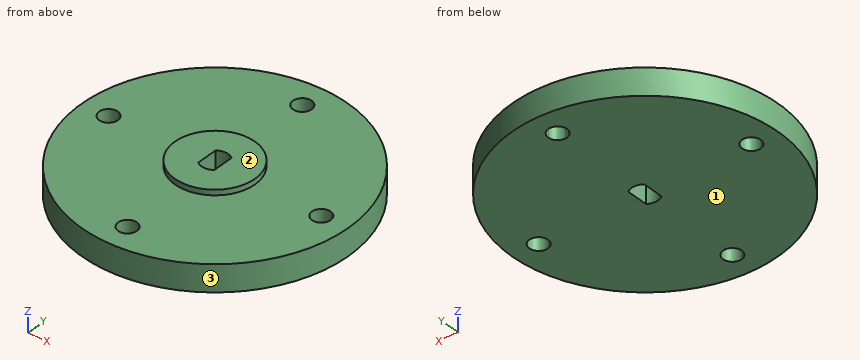
```python
from build123d import *

# Parameters (mm, degrees)
F0_R     = 7.5
F0_R_2   = 25
F1_DEPTH = 5
F2_DEPTH = 6
F3_R     = 1.75
F4_DEPTH = 5


with BuildPart() as f1:
    # F0 (on Top) → F1 (new body)
    with BuildSketch(Plane.XY):
        Circle(F0_R)
        with BuildLine():
            ThreePointArc((1.5, -2), (0, -2.5), (-1.5, -2))
            Line((-1.5, -2), (-1.5, 2))
            ThreePointArc((-1.5, 2), (0, 2.5), (1.5, 2))
            Line((1.5, 2), (1.5, -2))
        make_face(mode=Mode.SUBTRACT)
        Circle(F0_R_2)
        Circle(F0_R, mode=Mode.SUBTRACT)
    extrude(amount=F1_DEPTH)

    # F0 (on Top) → F2 (join)
    with BuildSketch(Plane.XY):
        Circle(F0_R)
        with BuildLine():
            ThreePointArc((1.5, -2), (0, -2.5), (-1.5, -2))
            Line((-1.5, -2), (-1.5, 2))
            ThreePointArc((-1.5, 2), (0, 2.5), (1.5, 2))
            Line((1.5, 2), (1.5, -2))
        make_face(mode=Mode.SUBTRACT)
    extrude(amount=F2_DEPTH)

    # F3 (on face) → F4 (cut)
    with BuildSketch(Plane.XY.offset(5)):
        with BuildLine():
            ThreePointArc((0, 18.25), (1.237437, 18.762563), (1.75, 20))
            ThreePointArc((1.75, 20), (-1.237437, 21.237437), (0, 18.25))
        make_face()
        with Locations((20, 0)):
            Circle(F3_R)
        with Locations((0, -20)):
            Circle(F3_R)
        with Locations((-20, 0)):
            Circle(F3_R)
    extrude(amount=-F4_DEPTH, mode=Mode.SUBTRACT)


solid = f1.part
```
Check sheet for the modelled part. Datum: model origin and axes. Units: mm. Face numbers are marked on the shaded views. Give positions to 0.01 mm unless a question says otherwise; leave off trailing zeros. Write each loop counter-clockwise with the first axis right and the second up, starting at its lowest first coordinate (ties: lowest second). Pieces come first, ordered by that corner, then holes.
Item 1: Draft check along Z on the marked faces 1, 2 and 3. Enter one of: released by +Z, released by -Z, zero draft, split by the parting line, or undercut.
Item 2: Scan lines: L1, parallel to Y at x = 0, z = 2.5; L2, parallel to Z at x = -5, y = 6.5; L3, parallel to X at y = 21.5, z = 2.4. Record each from-to range of solid material in increasing order.
Item 3: Cross-section at A-A (y = 0). Enter the section's corners in (x, z).
Item 4: Cross-section at B-B (x = -20). Enter the section's corners in (y, z).
Item 5: Cross-section at D-D (z = 1.1). Enter the section's corners in (x, y).
Item 6: Gauge pin test, flat ends, axial feed: pin 1 (1.5 mm diameter, centred on y = -8, z = 0.5, fed in from +X); pin 2 (4 mm diameter, centred on x = 0, y = -20, fed in from -Z); pin 3 (2 mm diameter, centred on x = 20, y = 0, fed in from -Z); pin 4 (1.5 mm diameter, centred on y = -17.5, z = 3.5, fed in from -X). Record the tip position at first contact, or that the pin passes through.
Report:
1. face 1: released by -Z
1. face 2: released by +Z
1. face 3: zero draft
2. L1: y = -25 to -21.75, -18.25 to -2.5, 2.5 to 18.25, 21.75 to 25
2. L2: z = 0 to 5
2. L3: x = -12.76 to -0.9, 0.9 to 12.76
3. outline: (-25, 0) - (-21.75, 0) - (-21.75, 5) - (-25, 5) - close; (-18.25, 0) - (-1.5, 0) - (-1.5, 6) - (-7.5, 6) - (-7.5, 5) - (-18.25, 5) - close; (1.5, 0) - (18.25, 0) - (18.25, 5) - (7.5, 5) - (7.5, 6) - (1.5, 6) - close; (21.75, 0) - (25, 0) - (25, 5) - (21.75, 5) - close
4. outline: (-15, 0) - (-1.75, 0) - (-1.75, 5) - (-15, 5) - close; (1.75, 0) - (15, 0) - (15, 5) - (1.75, 5) - close
5. outline: circle Ø50 at (0, 0); hole circle Ø3.5 at (-20, 0); hole circle Ø3.5 at (0, -20); hole circle Ø3.5 at (0, 20); hole (-1.5, -2) arc R2.5 ccw to (1.5, -2) - (1.5, 2) arc R2.5 ccw to (-1.5, 2) - close; hole circle Ø3.5 at (20, 0)
6. pin 1: stops at x = 23.93
6. pin 2: stops at z = 0
6. pin 3: passes through
6. pin 4: stops at x = -18.56
